from build123d import *

# Parameters (mm, degrees)
BOSS_EXTRUDE1_DEPTH = 1016


with BuildPart() as part:
    # Sketch1 → Boss-Extrude1 (new body)
    with BuildSketch(Plane.XY):
        with BuildLine():
            Line((-36.5, 14.096450845), (36.5, 14.096450845))
            Line((36.5, 14.096450845), (36.5, 8.496450845))
            Line((36.5, 8.496450845), (8.9, 8.496450845))
            ThreePointArc((8.9, 8.496450845), (3.950252532, 6.446198313), (1.9, 1.496450845))
            Line((1.9, 1.496450845), (1.9, -110.303549155))
            ThreePointArc((1.9, -110.303549155), (3.950252532, -115.253296624), (8.9, -117.303549155))
            Line((8.9, -117.303549155), (36.5, -117.303549155))
            Line((36.5, -117.303549155), (36.5, -122.903549155))
            Line((36.5, -122.903549155), (-36.5, -122.903549155))
            Line((-36.5, -122.903549155), (-36.5, -117.303549155))
            Line((-36.5, -117.303549155), (-8.9, -117.303549155))
            ThreePointArc((-8.9, -117.303549155), (-3.950252532, -115.253296624), (-1.9, -110.303549155))
            Line((-1.9, -110.303549155), (-1.9, 1.496450845))
            ThreePointArc((-1.9, 1.496450845), (-3.950252532, 6.446198313), (-8.9, 8.496450845))
            Line((-8.9, 8.496450845), (-36.5, 8.496450845))
            Line((-36.5, 8.496450845), (-36.5, 14.096450845))
        make_face()
    extrude(amount=BOSS_EXTRUDE1_DEPTH)


solid = part.part
The model under review builds one solid part; all positions refer to its coordinate system, in mm. A direction names the side the tool comes from. Give positions to 0.01 mm unless a question says otherwise; leave off trailing zeros. Order: outer loops, then holes, each group sorted by start corner. A loop starts at its lowest first (then second) coordinate and runs counter-clockwise, first axis right, second up. Notation, with made-up numbers: M 51,27.25 L 84,27.25 A20 ccw 84,42.25 Z; hole C 41,51 d4. An arc over 180 degrees is marked long. Answer in a Markdown table with one row per item. Add a question column.
1. Add section C-C on y = -56. State the section outline as (x, z) points.
2. Add section A-A on x = -28. State the section outline as (y, z) points, plus the area to 3 significant figures.
3. To check wall thickness, follow line 1 along Y through (x, z) = (31.5, 912.5); line 2 along X through (y, z) = (-38, 823); line 3 along Y through (x, z) = (8, 371). State the ranges of each line that lie inside material, in increasing order.
4. Mouldability with a two-part tool opening along Y and no side actions: class faces 1 (the flat face through (1, -122.904, 501)), 2 (the flat face through (0, -54, 1016)), 3 (the flat face through (-1, 14.096, 501)), 4 (the flat face through (-23, 8.496, 501)) as released by +Y, released by -Y, zero draft, split by the parting line, or undercut.
5. Add section B-B on z = 655.5. State the section outline as (x, y) points.
6. Machinability: for faces 5 (the flat face through (23, 8.496, 501)), 6 (the flat face through (-23, -117.304, 501)), 7 (the flat face through (0, -54, 0)), which of the approach directions +Z, -Z, +X, -X, +Y, -Y give a long, thin tool a straight path to every point of the face, cutting with its end or side? Answer none if there is none.
7. For pin 1 Ø10 at (x, y) = (8.5, -21) entering from +Z; pin 2 Ø12 at (y, z) = (-32, 794.5) entering from +X, all flat-tipped, find the tip position at first contact; note any pin that passes through.
The answers:
| question | item | result |
|---|---|---|
| 1 | outline | M -1.9,0 L 1.9,0 L 1.9,1016 L -1.9,1016 Z |
| 2 | outline | M -122.9,0 L -117.3,0 L -117.3,1016 L -122.9,1016 Z; M 8.5,0 L 14.1,0 L 14.1,1016 L 8.5,1016 Z |
| 2 | area | 11,400 mm2 |
| 3 | line 1 | -122.9 to -117.3, 8.5 to 14.1 |
| 3 | line 2 | -1.9 to 1.9 |
| 3 | line 3 | -122.9 to -117.25, 8.44 to 14.1 |
| 4 | face 1 | released by -Y |
| 4 | face 2 | zero draft |
| 4 | face 3 | released by +Y |
| 4 | face 4 | undercut |
| 5 | outline | M -36.5,-122.9 L 36.5,-122.9 L 36.5,-117.3 L 8.9,-117.3 A7 cw 1.9,-110.3 L 1.9,1.5 A7 cw 8.9,8.5 L 36.5,8.5 L 36.5,14.1 L -36.5,14.1 L -36.5,8.5 L -8.9,8.5 A7 cw -1.9,1.5 L -1.9,-110.3 A7 cw -8.9,-117.3 L -36.5,-117.3 Z |
| 6 | face 5 | +Z, -Z, +X |
| 6 | face 6 | +Z, -Z, -X |
| 6 | face 7 | -Z, +X, -X, +Y, -Y |
| 7 | pin 1 | through |
| 7 | pin 2 | x = 1.9 |
